Source: CAD feature listing. Evaluate the final solid. Frame: model axes, mm. Round coordinates to 2 decimals unless told otherwise and drop trailing zeros. Order: outer loops, then holes, each group sorted by start corner. A loop starts at its lowest first (then second) coordinate and runs counter-clockwise, first axis right, second up. Notation, with made-up numbers: M -35,37 L -29,37 A25 cw -29,68 Z; hole C 4,52 d8. An arc over 180 degrees is marked long. Use one line per item in the form item = value. Start each with the question number.
Q1. Section A-A (x = -74). Return the cut outline in (y, z) (3 decimals).
Q2. Material intervals for probe 1 along Y at (x, z) = (-59.5, 1.25) (3 decimals); probe 2 along Y at (x, z) = (0.5, 0); probe 3 along Z at (x, y) = (-15, -1), sorted ascending.
Q3. Contact query for flat-ended pins moving along their axis: pin 1 (4 mm diameter, centred on x = -46, y = -1, fed in from +Z); pin 2 (0.6 mm diameter, centred on y = 0.5, z = -1.5, fed in from +X); pin 3 (4 mm diameter, centred on x = 12.5, y = 1, fed in from -Z) (3 decimals). Output: stop coordinate, or through.
from build123d import *

# Parameters (mm, degrees)
SKETCH2_R                     = 9.525
BOSS_EXTRUDE1_DEPTH           = 3.175
BOSS_EXTRUDE1_TAPER           = 60
BOSS_EXTRUDE1_OTHER_WAY_DEPTH = 3.175
BOSS_EXTRUDE1_OTHER_WAY_TAPER = 60
BOSS_EXTRUDE2_DEPTH           = 2.38125
CUT_EXTRUDE1_DEPTH            = 90.465522276
CUT_EXTRUDE1_DEPTH_BACK       = 90.465522276
SKETCH5_W                     = 78.047666622
SKETCH5_H                     = 1.27
CUT_EXTRUDE2_DEPTH            = 1.27
SKETCH6_W                     = 78.047666622
SKETCH6_H                     = 1.27
CUT_EXTRUDE3_DEPTH            = 1.27
FILLET1_START                 = -88.9
FILLET1_DEPTH                 = 88.9
FILLET1_START_2               = -2.38125
FILLET1_2_DEPTH               = 4.7625
FILLET1_START_3               = -2.006559914
FILLET1_3_DEPTH               = 4.013119828


with BuildPart() as part:
    # Sketch1 → Revolve1 (revolve)
    with BuildSketch(Plane.XY, mode=Mode.PRIVATE) as revolve1_sk:
        with BuildLine():
            Line((0, 0), (0, 3.175))
            Line((0, 3.175), (1.587469063, 3.18491082))
            ThreePointArc((1.587469063, 3.18491082), (3.841885865, 2.257287955), (4.7625, 0))
            Line((4.7625, 0), (3.175, 0))
            Line((3.175, 0), (0, 0))
        make_face()
    revolve(revolve1_sk.sketch.rotate(Axis((-88.99, 0, 0), (1, 0, 0)), 90), axis=Axis((-88.99, 0, 0), (1, 0, 0)))

    # Sketch2 → Boss-Extrude1 (add)
    with BuildSketch(Plane.XY):
        with Locations((10.457777384, 0)):
            Circle(SKETCH2_R)
    extrude(amount=BOSS_EXTRUDE1_DEPTH, taper=BOSS_EXTRUDE1_TAPER)

    # Sketch2 → Boss-Extrude1 other way (add)
    with BuildSketch(Plane.XY):
        with Locations((10.457777384, 0)):
            Circle(SKETCH2_R)
    extrude(amount=-BOSS_EXTRUDE1_OTHER_WAY_DEPTH, taper=BOSS_EXTRUDE1_OTHER_WAY_TAPER)

    # Sketch3 → Boss-Extrude2 (add, symmetric)
    with BuildSketch(Plane.XY):
        Polygon((0, 2.006559914), (-88.9, 2.006559914), (-88.9, 0), (-88.9, -2.006559914), (0, -2.006559914), (0, 0), align=None)
    extrude(amount=BOSS_EXTRUDE2_DEPTH, both=True)

    # Sketch4 → Cut-Extrude1 (cut, two sides: drawn at the far end of the back side and taken through both)
    with BuildSketch(Plane(origin=(0, 0, 0), x_dir=(1, 0, 0), z_dir=(0, 1, 0)).offset(-CUT_EXTRUDE1_DEPTH_BACK)):
        Polygon((-82.55, 2.38125), (-81.847582607, 1.678832607), (-80.077417393, 1.678832607), (-79.375, 2.38125), align=None)
        Polygon((-80.077417393, -1.678832607), (-79.375, -2.38125), (-82.55, -2.38125), (-81.847582607, -1.678832607), align=None)
    extrude(amount=CUT_EXTRUDE1_DEPTH + CUT_EXTRUDE1_DEPTH_BACK, mode=Mode.SUBTRACT)

    # Sketch5 → Cut-Extrude2 (cut)
    with BuildSketch(Plane.XY.offset(2.38125)):
        with Locations((-39.023833311, 0)):
            Rectangle(SKETCH5_W, SKETCH5_H)
    extrude(amount=-CUT_EXTRUDE2_DEPTH, mode=Mode.SUBTRACT)

    # Sketch6 → Cut-Extrude3 (cut)
    with BuildSketch(Plane(origin=(0, 0, -2.38125), x_dir=(-1, 0, 0), z_dir=(0, 0, -1))):
        with Locations((39.023833311, 0)):
            Rectangle(SKETCH6_W, SKETCH6_H)
    extrude(amount=-CUT_EXTRUDE3_DEPTH, mode=Mode.SUBTRACT)

    # Fillet1: read off the stored shape, not the designer's step
    # Fillet1 outline → Fillet1 (cut)
    with BuildSketch(Plane.YZ.offset(FILLET1_START)):
        with BuildLine():
            Line((-2.006559914, 2.38125), (-2.006559914, 1.61925))
            ThreePointArc((-2.006559914, 1.61925), (-1.783375281, 2.158065367), (-1.244559914, 2.38125))
            Line((-1.244559914, 2.38125), (-2.006559914, 2.38125))
        make_face()
        with BuildLine():
            ThreePointArc((-1.244559914, -2.38125), (-1.783375281, -2.158065367), (-2.006559914, -1.61925))
            Line((-2.006559914, -1.61925), (-2.006559914, -2.38125))
            Line((-2.006559914, -2.38125), (-1.244559914, -2.38125))
        make_face()
        with BuildLine():
            Line((2.006559914, 2.38125), (1.244559914, 2.38125))
            ThreePointArc((1.244559914, 2.38125), (1.783375281, 2.158065367), (2.006559914, 1.61925))
            Line((2.006559914, 1.61925), (2.006559914, 2.38125))
        make_face()
        with BuildLine():
            ThreePointArc((2.006559914, -1.61925), (1.783375281, -2.158065367), (1.244559914, -2.38125))
            Line((1.244559914, -2.38125), (2.006559914, -2.38125))
            Line((2.006559914, -2.38125), (2.006559914, -1.61925))
        make_face()
    extrude(amount=FILLET1_DEPTH, mode=Mode.SUBTRACT)

    # Fillet1 2 outline → Fillet1 2 (cut)
    with BuildSketch(Plane.XY.offset(FILLET1_START_2)):
        with BuildLine():
            Line((-88.9, -2.006559914), (-88.138, -2.006559914))
            ThreePointArc((-88.138, -2.006559914), (-88.676815367, -1.783375281), (-88.9, -1.244559914))
            Line((-88.9, -1.244559914), (-88.9, -2.006559914))
        make_face()
        with BuildLine():
            Line((-88.9, 2.006559914), (-88.9, 1.244559914))
            ThreePointArc((-88.9, 1.244559914), (-88.676815367, 1.783375281), (-88.138, 2.006559914))
            Line((-88.138, 2.006559914), (-88.9, 2.006559914))
        make_face()
    extrude(amount=FILLET1_2_DEPTH, mode=Mode.SUBTRACT)

    # Fillet1 3 outline → Fillet1 3 (cut)
    with BuildSketch(Plane(origin=(0, 0, 0), x_dir=(1, 0, 0), z_dir=(0, 1, 0)).offset(FILLET1_START_3)):
        with BuildLine():
            ThreePointArc((-88.138, -2.38125), (-88.676815367, -2.158065367), (-88.9, -1.61925))
            Line((-88.9, -1.61925), (-88.9, -2.38125))
            Line((-88.9, -2.38125), (-88.138, -2.38125))
        make_face()
        with BuildLine():
            Line((-88.9, 2.38125), (-88.9, 1.61925))
            ThreePointArc((-88.9, 1.61925), (-88.676815367, 2.158065367), (-88.138, 2.38125))
            Line((-88.138, 2.38125), (-88.9, 2.38125))
        make_face()
    extrude(amount=FILLET1_3_DEPTH, mode=Mode.SUBTRACT)


solid = part.part
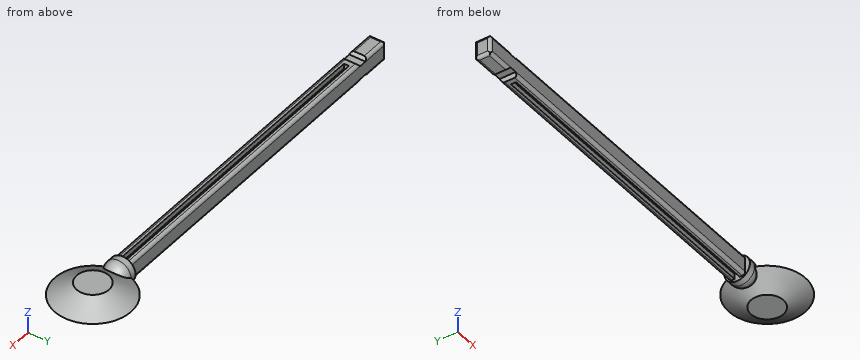
Results list:
q1.outline = M -2.007,-1.619 A0.762 ccw -1.245,-2.381 L -0.635,-2.381 L -0.635,-1.111 L 0.635,-1.111 L 0.635,-2.381 L 1.245,-2.381 A0.762 ccw 2.007,-1.619 L 2.007,1.619 A0.762 ccw 1.245,2.381 L 0.635,2.381 L 0.635,1.111 L -0.635,1.111 L -0.635,2.381 L -1.245,2.381 A0.762 ccw -2.007,1.619 Z
q2.probe_1 = -2.007 to -0.635, 0.635 to 2.007
q2.probe_2 = -3.18 to 3.18
q2.probe_3 = -2.38 to 2.38
q3.pin_1 = 2.38
q3.pin_2 = 17.89
q3.pin_3 = -3.175
